Design review of the part built by this model. Coordinates are the model's own, in mm. Face numbers are marked on the shaded views. A direction names the side the tool comes from. Round coordinates to 2 decimals unless told otherwise and drop trailing zeros. Write each loop counter-clockwise with the first axis right and the second up, starting at its lowest first coordinate (ties: lowest second). Pieces come first, ordered by that corner, then holes. Notation, with made-up numbers: (16, 88.25) - (53, 88.25) arc R12 ccw to (53, 107.25) - close; hole circle Ø4 at (36, 40). An arc over 180 degrees is marked (long way). Use one line per item in the form item = value.
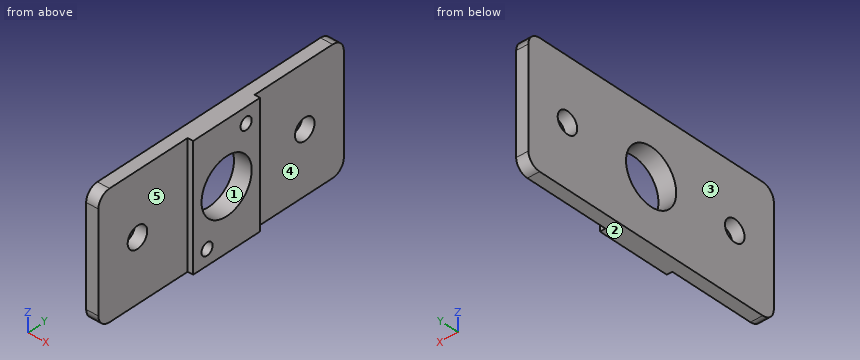
```python
from build123d import *

# Parameters (mm, degrees)
BOSS_EXTRUDE1_DEPTH = 20
SKETCH2_R           = 1.75
SKETCH2_R_2         = 4.5
CUT_EXTRUDE1_DEPTH  = 3.9
SKETCH3_R           = 1
CUT_EXTRUDE2_DEPTH  = 1.8
FILLET1_R           = 2


with BuildPart() as part:
    # Sketch1 → Boss-Extrude1 (new body)
    with BuildSketch(Plane.XY):
        Polygon((0, 0), (0, -44), (2, -44), (2, -28), (2.9, -28), (2.9, -16), (2, -16), (2, 0), align=None)
    extrude(amount=BOSS_EXTRUDE1_DEPTH)

    # Sketch2 → Cut-Extrude1 (cut, through all)
    with BuildSketch(Plane.ZY):
        with Locations((10, -7)):
            Circle(SKETCH2_R)
        with Locations((10, -37)):
            Circle(SKETCH2_R)
        with Locations((10, -22)):
            Circle(SKETCH2_R_2)
    extrude(amount=-CUT_EXTRUDE1_DEPTH, mode=Mode.SUBTRACT)

    # Sketch3 → Cut-Extrude2 (cut)
    with BuildSketch(Plane(origin=(2.9, 0, 0), x_dir=(0, 0, -1), z_dir=(1, 0, 0))):
        with Locations((-17.5, -18.5)):
            Circle(SKETCH3_R)
        with Locations((-2.5, -25.5)):
            Circle(SKETCH3_R)
    extrude(amount=-CUT_EXTRUDE2_DEPTH, mode=Mode.SUBTRACT)

    # Fillet1
    fillet1_edges = [part.edges().sort_by_distance(p)[0] for p in [
        (1, -44, 20),
        (1, 0, 0),
        (1, 0, 20),
        (1, -44, 0),
    ]]
    fillet(fillet1_edges, radius=FILLET1_R)


solid = part.part
```
Q1. We need section D-D on z = 2.5. Write out the cut boundary in (x, y), then the cut area to 3 significant figures.
Calculated:
outline = (0, -44) - (2, -44) - (2, -28) - (2.9, -28) - (2.9, -26.5) - (1.1, -26.5) - (1.1, -24.5) - (2.9, -24.5) - (2.9, -16) - (2, -16) - (2, 0) - (0, 0) - close
area = 95.2 mm2
Q2. We need section B-B on x = 0.6. Write out the cut boundary in (y, z).
Calculated:
outline = (-44, 2) arc R2 ccw to (-42, 0) - (-2, 0) arc R2 ccw to (0, 2) - (0, 18) arc R2 ccw to (-2, 20) - (-42, 20) arc R2 ccw to (-44, 18) - close; hole circle Ø3.5 at (-37, 10); hole circle Ø9 at (-22, 10); hole circle Ø3.5 at (-7, 10)
Q3. For P1, Ø10, axis at y = -29, z = 13.5, coming from the -X side; P2, Ø8, axis at y = -10.5, z = 5.5, coming from the +X side; P3, Ø3, axis at y = -37, z = 10, coming from the +X side; P4, Ø0.6, axis at y = -18, z = 17.5, coming from the +X side, all flat-tipped, find the tip position at first contact; note any pin that passes through.
Calculated:
P1 = 0
P2 = 2
P3 = through
P4 = 1.1
Q4. Machinability: for the marked faces 3, 4 and 5, which of the approach directions +Z, -Z, +X, -X, +Y, -Y give a long, thin tool a straight path to every point of the face, cutting with its end or side? Answer none if there is none.
Calculated:
face_3 = +Z, -Z, -X, +Y, -Y
face_4 = +Z, -Z, +X, +Y
face_5 = +Z, -Z, +X, -Y
Q5. We need section A-A on y = -22. Write out the cut boundary in (x, z).
Calculated:
outline = (0, 0) - (2.9, 0) - (2.9, 5.5) - (0, 5.5) - close; (0, 14.5) - (2.9, 14.5) - (2.9, 20) - (0, 20) - close
Q6. Draft analysis for pull direction Y (two halves, no side actions). For the marked faces 1 and 2, state which applies: released by +Y, released by -Y, zero draft, split by the parting line, or undercut.
Calculated:
face_1 = undercut
face_2 = zero draft
Q7. We need section C-C on y = -37. Write out the cut boundary in (x, z).
Calculated:
outline = (0, 0) - (2, 0) - (2, 8.25) - (0, 8.25) - close; (0, 11.75) - (2, 11.75) - (2, 20) - (0, 20) - close
Q8. To check wall thickness, follow line 1 along Y through (x, z) = (0.65, 10); line 2 along Y through (x, z) = (1.5, 17.5); line 3 along Y through (x, z) = (1.8, 14). State the ranges of each line that lie inside material, in increasing order. Write a range as from..to.
Calculated:
line_1 = -44..-38.75, -35.25..-26.5, -17.5..-8.75, -5.25..0
line_2 = -44..-19.5, -17.5..0
line_3 = -44..-24.06, -19.94..0
